Check sheet for the drawn part. Datum: minimum x, y, z corner. Units: mm. Round coordinates to 2 decimals unless told otherwise and drop trailing zeros. Order: outer loops, then holes, each group sorted by start corner. A loop starts at its lowest first (then second) coordinate and runs counter-clockwise, first axis right, second up. Notation, with made-up numbers: M -28.75,22 L -1.75,22 A19 ccw -1.75,42 Z; hole C 11,-3 d8. An arc over 180 degrees is marked long. Use one line per item in the form item = value. Start each with the question number.
Item 1: Cross-section at D-D on x = 37. Enter the section's corners in (y, z).
Item 2: Cross-section at A-A on x = 5.5. Enter the section's corners in (y, z).
Item 3: Go/stop test with flat-tipped pins: pin 1 Ø0.7 at (y, z) = (1.5, 12) entering from -X; pin 2 Ø0.8 at (x, y) = (43, 0.5) entering from -Z; pin 3 Ø0.7 at (y, z) = (1.5, 11) entering from +X; pin 4 Ø1.5 at (y, z) = (1.5, 6) entering from -X. Record where each tip stops, or that it passes through.
Item 4: Cross-section at B-B on x = 29. Enter the section's corners in (y, z), then the cut area to 3 significant figures.
Item 5: Thickness scan on probe 1 along Z at (x, y) = (7.5, 0.5); probe 2 along Y at (x, z) = (46.5, 5.75); probe 3 along Z at (x, y) = (23, 2.2). Record the ranges inside material, lowest first. Write a range as [from, to].
Item 6: Cross-section at C-C on z = 12. Enter the section's corners in (x, y).
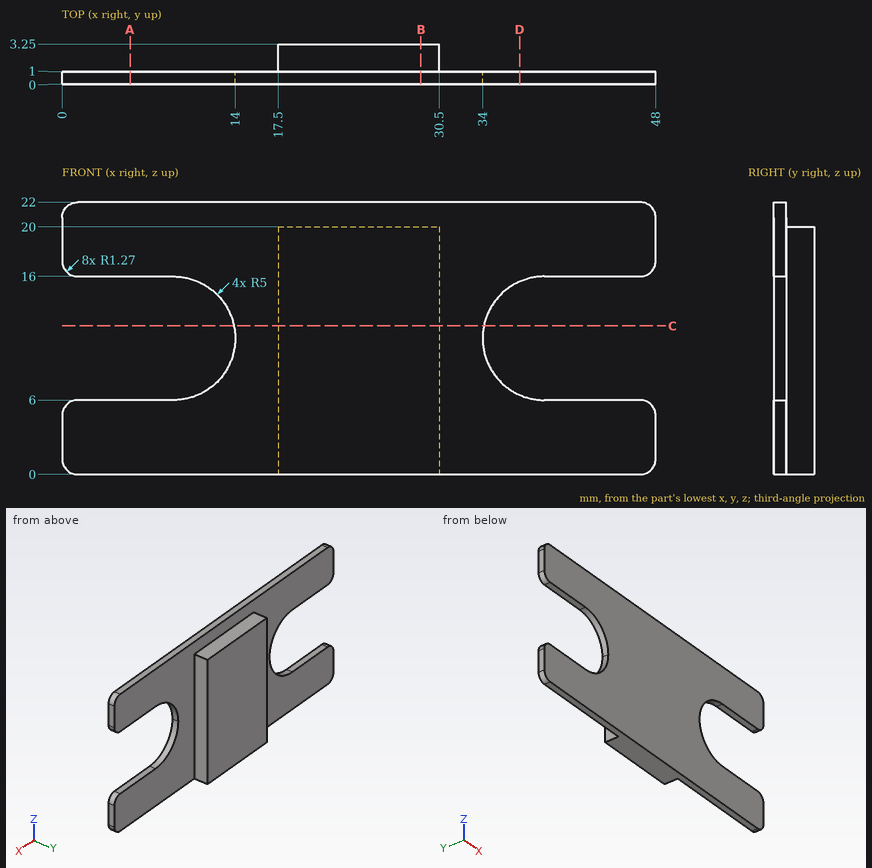
Output values:
q1.outline = M 0,0 L 1,0 L 1,6.42 L 0,6.42 Z; M 0,15.58 L 1,15.58 L 1,22 L 0,22 Z
q2.outline = M 0,0 L 1,0 L 1,6 L 0,6 Z; M 0,16 L 1,16 L 1,22 L 0,22 Z
q3.pin_1 = 17.5
q3.pin_2 = 0
q3.pin_3 = 30.5
q3.pin_4 = 0.22
q4.outline = M 0,0 L 3.25,0 L 3.25,20 L 1,20 L 1,22 L 0,22 Z
q4.area = 67.0 mm2
q5.probe_1 = [0, 6], [16, 22]
q5.probe_2 = [0, 1]
q5.probe_3 = [0, 20]
q6.outline = M 13.9,0 L 34.1,0 L 34.1,1 L 30.5,1 L 30.5,3.25 L 17.5,3.25 L 17.5,1 L 13.9,1 Z
